```python
from build123d import *

# Parameters (mm, degrees)
SKETCH1_W                = 74.549
SKETCH1_H                = 74.549
SKETCH1_R                = 26.67
BOSS_EXTRUDE1_DEPTH      = 1.27
BOSS_EXTRUDE1_DEPTH_BACK = 1.27
SKETCH2_R                = 3.302
CUT_EXTRUDE1_DEPTH       = 3.54
MIRROR2_COPY_1_SKETCH_R  = 3.302
MIRROR2_COPY_1_DEPTH     = 3.54
SKETCH14_OUTSIDE_W       = 97.642
SKETCH14_OUTSIDE_H       = 97.642
SKETCH14_OUTSIDE_R       = 34.798
CUT_EXTRUDE6_DEPTH       = 3.54


with BuildPart() as part:
    # Sketch1 → Boss-Extrude1 (new body, two sides)
    with BuildSketch(Plane.XY) as boss_extrude1_sk:
        Rectangle(SKETCH1_W, SKETCH1_H)
        Circle(SKETCH1_R, mode=Mode.SUBTRACT)
    extrude(amount=BOSS_EXTRUDE1_DEPTH)
    extrude(boss_extrude1_sk.sketch, amount=-BOSS_EXTRUDE1_DEPTH_BACK)

    # Sketch2 → Cut-Extrude1 (cut, through all)
    with BuildSketch(Plane.XY.offset(1.27)):
        with Locations((-31.75, 31.75)):
            Circle(SKETCH2_R)
    cut_extrude1 = extrude(amount=-CUT_EXTRUDE1_DEPTH, mode=Mode.SUBTRACT)

    # Mirror1: Cut-Extrude1 across plane
    add(cut_extrude1.mirror(Plane(origin=(0, 0, 0), x_dir=(0, 0, 1), z_dir=(1, 0, 0))), mode=Mode.SUBTRACT)

    # Mirror2: Cut-Extrude1 across plane
    add(cut_extrude1.mirror(Plane.ZX), mode=Mode.SUBTRACT)

    # Mirror2 copy 1 sketch → Mirror2 copy 1 (cut, through all)
    with BuildSketch(Plane(origin=(0, 0, 1.27), x_dir=(-1, 0, 0), z_dir=(0, 0, 1))):
        with Locations((-31.75, 31.75)):
            Circle(MIRROR2_COPY_1_SKETCH_R)
    extrude(amount=-MIRROR2_COPY_1_DEPTH, mode=Mode.SUBTRACT)

    # Sketch14 outside → Cut-Extrude6 (cut, through all)
    with BuildSketch(Plane.XY.offset(1.27)):
        Rectangle(SKETCH14_OUTSIDE_W, SKETCH14_OUTSIDE_H)
        Circle(SKETCH14_OUTSIDE_R, mode=Mode.SUBTRACT)
    extrude(amount=-CUT_EXTRUDE6_DEPTH, mode=Mode.SUBTRACT)


solid = part.part
```
Build history of the part. All positions in model axes, mm. Coordinates: 2 decimals unless noted, no trailing zeros. Write each loop counter-clockwise with the first axis right and the second up, starting at its lowest first coordinate (ties: lowest second). Pieces come first, ordered by that corner, then holes.
1. Band-saw the part on C-C, the plane z = -0.45. Give the cut face in (x, y), and give its area (3 significant figures).
Answer block:
outline: circle Ø69.6 at (0, 0); hole circle Ø53.34 at (0, 0)
area: 1,570 mm2
2. Band-saw the part on A-A, the plane x = 0. Give the cut face in (y, z), and give its area (3 significant figures).
Answer block:
outline: (-34.8, -1.27) - (-26.67, -1.27) - (-26.67, 1.27) - (-34.8, 1.27) - close; (26.67, -1.27) - (34.8, -1.27) - (34.8, 1.27) - (26.67, 1.27) - close
area: 41.3 mm2
3. Drop flat-ended pins along their axis: pin 1 (1.5 mm diameter, centred on x = 2.5, z = 0.5, fed in from +Y); pin 2 (1 mm diameter, centred on x = -25, z = 0, fed in from -Y); pin 3 (6 mm diameter, centred on x = -16.5, y = 15.5, fed in from +Z). Give the stop position or say it passes through.
Answer block:
pin 1: stops at y = 34.75
pin 2: stops at y = -24.71
pin 3: passes through
4. Drill centre lines: probe 1 along Y at (x, z) = (-24, -0.3); probe 2 along Y at (x, z) = (0, -0.95). Where is each one in solid material? Low to high.
Answer block:
probe 1: y = -25.2 to -11.63, 11.63 to 25.2
probe 2: y = -34.8 to -26.67, 26.67 to 34.8
